```python
from build123d import *

# Parameters (mm, degrees)
SKETCH_1_W          = 64
SKETCH_1_H          = 82
SKETCH_1_R          = 1.25
EXTRUDE_1_DEPTH     = 2
FILLET_1_R          = 3
SKETCH_3_R          = 1.515
CUT_EXTRUDE_1_DEPTH = 10
CUT_EXTRUDE_2_DEPTH = 10
FILLET_2_R          = 1.5


with BuildPart() as part:
    # 草图1 → 凸台-拉伸1 (new body)
    with BuildSketch(Plane.XY):
        Rectangle(SKETCH_1_W, SKETCH_1_H)
        with Locations((-27, 36)):
            Circle(SKETCH_1_R, mode=Mode.SUBTRACT)
        with Locations((27, 36)):
            Circle(SKETCH_1_R, mode=Mode.SUBTRACT)
        with Locations((27, -36)):
            Circle(SKETCH_1_R, mode=Mode.SUBTRACT)
        with Locations((-27, -36)):
            Circle(SKETCH_1_R, mode=Mode.SUBTRACT)
    extrude(amount=EXTRUDE_1_DEPTH)

    # 圆角1
    fillet_1_edges = [part.edges().sort_by_distance(p)[0] for p in [
        (32, -41, 1),
        (-32, -41, 1),
        (-32, 41, 1),
        (32, 41, 1),
    ]]
    fillet(fillet_1_edges, radius=FILLET_1_R)

    # 草图3 → 切除-拉伸1 (cut)
    with BuildSketch(Plane.XY.offset(2)):
        with Locations((-26, 15)):
            Circle(SKETCH_3_R)
        with Locations((-26, -5)):
            Circle(SKETCH_3_R)
        with Locations(Location((26, -5, 0), (0, 0, 180))):
            Circle(SKETCH_3_R)
        with Locations(Location((26, 15, 0), (0, 0, 180))):
            Circle(SKETCH_3_R)
    extrude(amount=-CUT_EXTRUDE_1_DEPTH, mode=Mode.SUBTRACT)

    # 草图4 → 切除-拉伸2 (cut)
    with BuildSketch(Plane.XY.offset(2)):
        Polygon((-23, 29.53728915), (-23, -29.53728915), (-3.589781416, 0), align=None)
        Polygon((-19.410218584, 35), (0, 5.46271085), (19.410218584, 35), align=None)
        Polygon((23, 29.53728915), (3.589781416, 0), (23, -29.53728915), align=None)
        Polygon((0, -5.46271085), (-19.410218584, -35), (19.410218584, -35), align=None)
    extrude(amount=-CUT_EXTRUDE_2_DEPTH, mode=Mode.SUBTRACT)

    # 圆角2
    fillet_2_edges = [part.edges().sort_by_distance(p)[0] for p in [
        (0, -5.46271085, 1),
        (19.410218584, -35, 1),
        (-19.410218584, -35, 1),
        (-23, 29.53728915, 1),
        (-3.589781416, 0, 1),
        (-23, -29.53728915, 1),
        (3.589781416, 0, 1),
        (23, 29.53728915, 1),
        (23, -29.53728915, 1),
        (-19.410218584, 35, 1),
        (19.410218584, 35, 1),
        (0, 5.46271085, 1),
    ]]
    fillet(fillet_2_edges, radius=FILLET_2_R)


solid = part.part
```
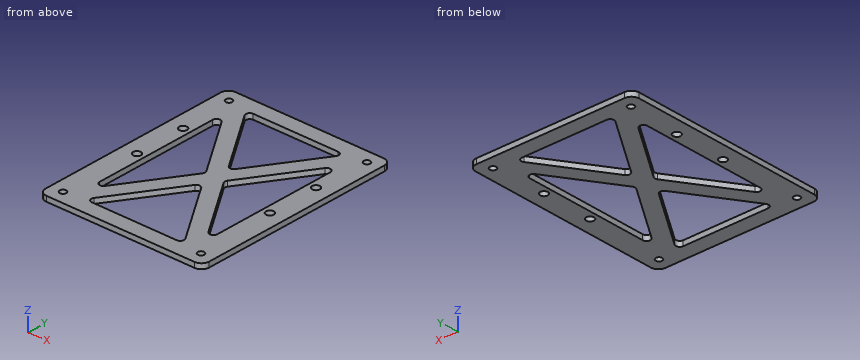
Could you check a few things on this model? Use its own coordinates, in mm. Give positions to 0.01 mm unless a question says otherwise; leave off trailing zeros. Loops run counter-clockwise (first coordinate to the right, second up) from the corner with the lowest first, then second, coordinate; pieces in that order, holes last. Notation, with made-up numbers: (24, 42.5) -> (72, 42.5) arc R23 ccw to (72, 80.5) -> close; hole circle Ø4 at (22, 55). An arc over 180 degrees is marked (long way). Put each result on its own line as item: value.
(1) Imagine slicing it at D-D on x = -14.5. Write out the boundary of the cut face in (y, z), plus the area to 3 significant figures.
Computed:
outline: (-41, 0) -> (-35, 0) -> (-35, 2) -> (-41, 2) -> close; (-27.53, 0) -> (-16.6, 0) -> (-16.6, 2) -> (-27.53, 2) -> close; (16.6, 0) -> (27.53, 0) -> (27.53, 2) -> (16.6, 2) -> close; (35, 0) -> (41, 0) -> (41, 2) -> (35, 2) -> close
area: 67.7 mm^2
(2) Imagine slicing it at A-A on y = 36. Write out the boundary of the cut face in (x, z), plus the area to 3 significant figures.
Computed:
outline: (-32, 0) -> (-28.25, 0) -> (-28.25, 2) -> (-32, 2) -> close; (-25.75, 0) -> (25.75, 0) -> (25.75, 2) -> (-25.75, 2) -> close; (28.25, 0) -> (32, 0) -> (32, 2) -> (28.25, 2) -> close
area: 118 mm^2
(3) Imagine slicing it at C-C on y = -5. Write out the boundary of the cut face in (x, z) (1 decimal), plus the area to 3 significant figures.
Computed:
outline: (-32, 0) -> (-27.5, 0) -> (-27.5, 2) -> (-32, 2) -> close; (-24.5, 0) -> (-23, 0) -> (-23, 2) -> (-24.5, 2) -> close; (-6.9, 0) -> (6.9, 0) -> (6.9, 2) -> (-6.9, 2) -> close; (23, 0) -> (24.5, 0) -> (24.5, 2) -> (23, 2) -> close; (27.5, 0) -> (32, 0) -> (32, 2) -> (27.5, 2) -> close
area: 51.4 mm^2
(4) Please list where these lines run through material, in increasing order: probe 1 along X at (y, z) = (-6, 0.5); probe 2 along Y at (x, z) = (-15.5, 0.6); probe 3 along X at (y, z) = (-18.5, 1.7). Write a range as [from, to].
Computed:
probe 1: [-32, -27.14], [-24.86, -23], [-7.53, 7.53], [23, 24.86], [27.14, 32]
probe 2: [-41, -35], [-29.05, -18.12], [18.12, 29.05], [35, 41]
probe 3: [-32, -23], [-15.75, -8.57], [8.57, 15.75], [23, 32]
(5) Imagine slicing it at B-B on x = -21.5. Write out the boundary of the cut face in (y, z), plus the area to 3 significant figures.
Computed:
outline: (-41, 0) -> (-26.02, 0) -> (-26.02, 2) -> (-41, 2) -> close; (26.02, 0) -> (41, 0) -> (41, 2) -> (26.02, 2) -> close
area: 59.9 mm^2
